Source: CAD feature listing. Evaluate the final solid. Frame: model axes, mm. Coordinates: 2 decimals unless noted, no trailing zeros. Order: outer loops, then holes, each group sorted by start corner. A loop starts at its lowest first (then second) coordinate and runs counter-clockwise, first axis right, second up. Notation, with made-up numbers: (-22, 21) -> (19, 21) arc R27 ccw to (19, 52) -> close; hole circle Ø10 at (81, -33). An arc over 180 degrees is marked (long way). Put each result on its own line as item: value.
from build123d import *

# Parameters (mm, degrees)
F1_DEPTH = 25


with BuildPart() as f1:
    # F0 (on Front) → F1 (new body)
    with BuildSketch(Plane.XZ):
        with BuildLine():
            ThreePointArc((34.060664, -32.569028), (43.737952, -17.545993), (47.126111, 0))
            ThreePointArc((47.126111, 0), (43.334293, 18.520512), (32.569028, 34.060664))
            Line((32.569028, 34.060664), (0, 0))
            Line((0, 0), (34.060664, -32.569028))
        make_face()
        with BuildLine():
            Line((0, 0), (32.569028, 34.060664))
            ThreePointArc((32.569028, 34.060664), (1.069264, 47.113979), (-30.990258, 35.503158))
            Line((-30.990258, 35.503158), (0, 0))
        make_face()
        with BuildLine():
            ThreePointArc((-35.503158, -30.990258), (-1.069264, -47.113979), (34.060664, -32.569028))
            Line((34.060664, -32.569028), (0, 0))
            Line((0, 0), (-35.503158, -30.990258))
        make_face()
        with BuildLine():
            Line((0, 0), (-30.990258, 35.503158))
            ThreePointArc((-30.990258, 35.503158), (-47.017946, 3.191102), (-35.503158, -30.990258))
            Line((-35.503158, -30.990258), (0, 0))
        make_face()
    extrude(amount=F1_DEPTH)


solid = f1.part
1. First-contact query: pin 1 (5 mm diameter, centred on x = 9.5, y = -8, fed in from +Z); pin 2 (2 mm diameter, centred on y = -9.5, z = -35, fed in from -X); pin 3 (5 mm diameter, centred on x = 16, y = -21.5, fed in from -Z). Flat tips, straight axial feed; report the tip coordinate or a pass-through.
Numbers:
pin 1: stops at z = 46.6
pin 2: stops at x = -32.63
pin 3: stops at z = -45.15
2. Cut plane C-C on z = 41.5. Output: boundary loops of the cut face in (x, y), plus the area to 3 significant figures.
Numbers:
outline: (-22.33, -25) -> (22.33, -25) -> (22.33, 0) -> (-22.33, 0) -> close
area: 1,120 mm2
3. Cut plane A-A on y = -9.5. Output: boundary loops of the cut face in (x, z).
Numbers:
outline: (-35.5, -30.99) arc R47.13 ccw to (34.06, -32.57) arc R47.13 ccw to (47.13, 0) arc R47.13 ccw to (32.57, 34.06) arc R47.13 ccw to (-30.99, 35.5) arc R47.13 ccw to start
4. Cut plane B-B on x = -26.5. Output: boundary loops of the cut face in (y, z), plus the area to 3 significant figures.
Numbers:
outline: (-25, -38.97) -> (0, -38.97) -> (0, 38.97) -> (-25, 38.97) -> close
area: 1,950 mm2
5. Ray query, line 1 along X through (y, z) = (-3, -31); line 2 along X through (y, z) = (-3.25, -6); line 3 along Z through (x, y) = (-16, -14.25). Return the intervals inside material, ascending.
Numbers:
line 1: x = -35.49 to 35.49
line 2: x = -46.74 to 46.74
line 3: z = -44.33 to 44.33
